For this review, use the dimensioned drawing (mm, ordinates from the lowest corner) and the shaded views. Round coordinates to 2 decimals unless told otherwise and drop trailing zeros. Write each loop counter-clockwise with the first axis right and the second up, starting at its lowest first coordinate (ties: lowest second). Pieces come first, ordered by that corner, then holes. Notation, with made-up numbers: (-32.5, 26.25) - (-17.5, 26.25) arc R16 ccw to (-17.5, 49.25) - close; hole circle Ø4 at (71, 50.5). An arc over 180 degrees is marked (long way). Write each question's results on one line, items separated by ' | '.
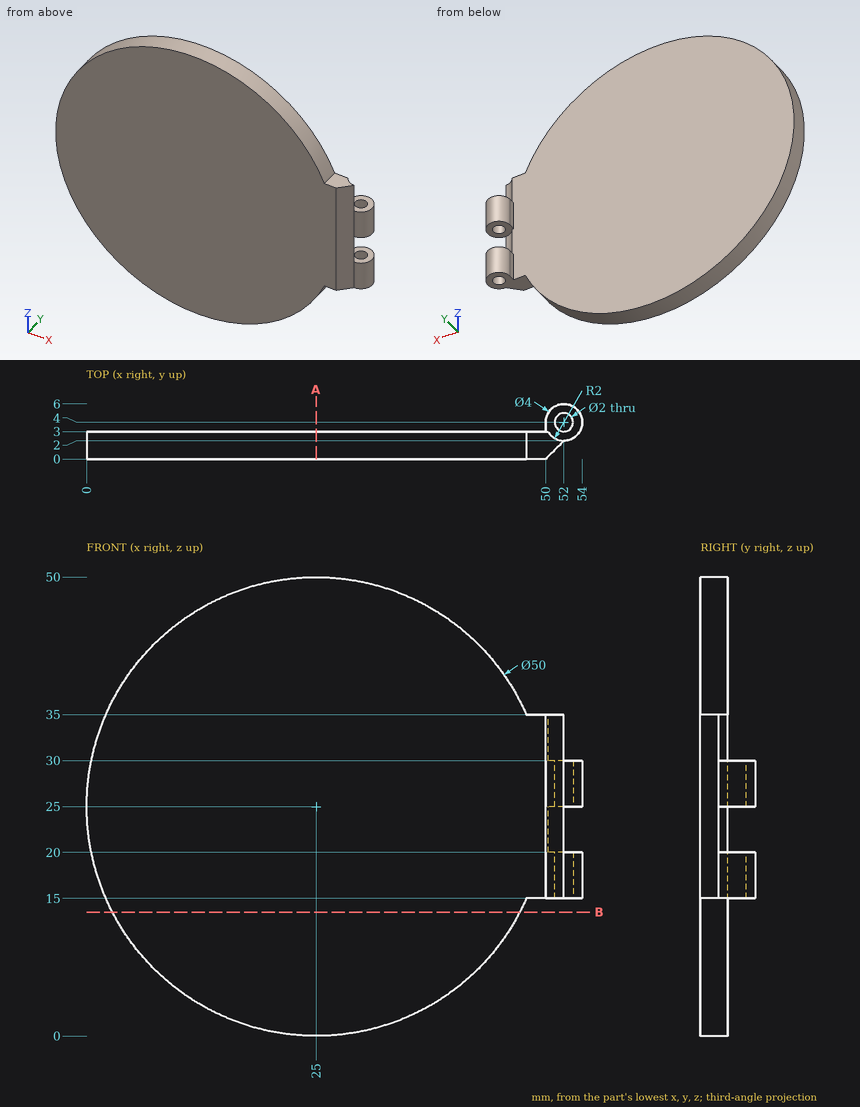
Q1. For probe 1 along Y at (x, z) = (52, 17); probe 2 along Y at (x, z) = (24, 40); probe 3 along Z at (x, y) = (51, 2.05), list the stretches that pass through material, from the lowest coordinate up.
Evaluation:
probe 1: y = 2 to 3, 5 to 6 | probe 2: y = 0 to 3 | probe 3: z = 15 to 35
Q2. Insertion check: P1, Ø25, axis at x = 13.5, z = 28.5, coming from the +Y side; P2, Ø1.8, axis at x = 50, y = 3.5, coming from the -Z side; P3, Ø1.2, axis at x = 53, y = 4.5, coming from the +Z side. Each pin has a flat end and moves straight along its axis. Give the tip position at first contact, or say it passes through.
Evaluation:
P1: stops at y = 3 | P2: stops at z = 15 | P3: stops at z = 30
Q3. We need section A-A (x = 25). State the section outline as (y, z) points, plus the area to 3 significant figures.
Evaluation:
outline: (0, 0) - (3, 0) - (3, 50) - (0, 50) - close | area: 150 mm^2
Q4. We need section B-B (z = 13.5). State the section outline as (x, y) points, plus the area to 3 significant figures.
Evaluation:
outline: (2.8, 0) - (47.2, 0) - (47.2, 3) - (2.8, 3) - close | area: 133 mm^2
